Part model, mm, in its own coordinate system. A direction names the side the tool comes from. Coordinates: 2 decimals unless noted, no trailing zeros. Loops run counter-clockwise (first coordinate to the right, second up) from the corner with the lowest first, then second, coordinate; pieces in that order, holes last. Notation, with made-up numbers: (-0.5, 67.5) - (25.5, 67.5) arc R17 ccw to (25.5, 74.5) - close; hole circle Ø9 at (23.25, 54). An arc over 180 degrees is marked (long way). Use a Markdown table: item, result. Add a question column.
1) Band-saw the part on A-A (y = 2.55). Give the cut face in (x, z).
2) Band-saw the part on D-D (x = 24). Give the cut face in (y, z).
3) Pull direction X, two halves, no side cores. Call faces 4 (the face through (31, 5, -8)), 5 (the face through (67.47, 2.54, -27.45)), 6 (the face through (4.5, 2, -5)): +X half, -X half, draft (parallel to the pull), parting line (faces both ways), or undercut.
4) Band-saw the part on B-B (z = -20.5). Give the cut face in (x, y).
5) Probe probe 1 along X at (y, z) = (2.85, 0); probe 2 along X at (y, z) = (3.5, -10.5); probe 3 along X at (y, z) = (3.9, -18). List the from-to ranges inside material, lowest first. Write a range as [from, to].
6) Drop flat-ended pins along their axis: P1, Ø3, axis at x = 32, y = 3.5, coming from the -Z side; P2, Ø1, axis at x = 5.5, y = 2.5, coming from the +Z side. Give the stop position or say it passes through.
7) Band-saw the part on C-C (x = 64). Give the cut face in (y, z), plus the area to 3 significant figures.
8) Tool access for faces 1 (the face through (62.137, 2.465, 0.969)), 2 (the face through (59.5, 2, -6)), 3 (the face through (58.68, 2.46, -22.93)): list every direction of +Z, -Z, +X, -X, +Y, -Y with a clear straight run to the whole face (end or side of a thin tool).
from build123d import *

# Parameters (mm, degrees)
SKETCH1_R           = 2.1
BOSS_EXTRUDE1_DEPTH = 5
FILLET2_R           = 2


with BuildPart() as part:
    # Sketch1 → Boss-Extrude1 (new body)
    with BuildSketch(Plane(origin=(0, 0, 0), x_dir=(1, 0, 0), z_dir=(0, 1, 0))):
        with BuildLine():
            Line((68.5, 0), (68.5, 15))
            Line((68.5, 15), (68.5, 24.639286301))
            Line((68.5, 24.639286301), (68.5, 29.417680708))
            Line((68.5, 29.417680708), (51.680517538, 18.308520556))
            ThreePointArc((51.680517538, 18.308520556), (31.678817451, 11.020026075), (11.677117365, 18.308520556))
            Line((11.677117365, 18.308520556), (-4.5, 28.993402687))
            Line((-4.5, 28.993402687), (-4.5, 0))
            ThreePointArc((-4.5, 0), (0, -4.5), (4.5, 0))
            Line((4.5, 0), (4.5, 15))
            ThreePointArc((4.5, 15), (32, 5.201587921), (59.5, 15))
            Line((59.5, 15), (59.5, 0))
            ThreePointArc((59.5, 0), (64, -4.5), (68.5, 0))
        make_face()
        with Locations(Location((0, 0, 0), (0, 0, 270))):
            Circle(SKETCH1_R, mode=Mode.SUBTRACT)
        with Locations(Location((64, 0, 0), (0, 0, 270))):
            Circle(SKETCH1_R, mode=Mode.SUBTRACT)
    extrude(amount=BOSS_EXTRUDE1_DEPTH)

    # Fillet2
    fillet2_edges = [part.edges().sort_by_distance(p)[0] for p in [
        (59.5, 2.5, -15),
        (4.5, 2.5, -15),
        (-4.5, 2.5, -28.993402687),
        (11.677117365, 2.5, -18.308520556),
        (51.680517538, 2.5, -18.308520556),
        (68.5, 2.5, -29.417680708),
    ]]
    fillet(fillet2_edges, radius=FILLET2_R)


solid = part.part
Answer block:
| question | item | result |
|---|---|---|
| 1 | outline | (-4.5, -25.28) arc R2 ccw to (-1.4, -26.94) - (11.58, -18.37) arc R2 ccw to (11.76, -18.24) arc R31.09 cw to (51.6, -18.24) arc R2 ccw to (51.78, -18.37) - (65.4, -27.37) arc R2 ccw to (68.5, -25.7) - (68.5, 0) arc R4.5 ccw to (59.5, 0) - (59.5, -11.02) arc R2 cw to (56.38, -12.68) arc R43.49 ccw to (7.62, -12.68) arc R2 cw to (4.5, -11.02) - (4.5, 0) arc R4.5 ccw to (-4.5, 0) - close; hole circle Ø4.2 at (0, 0); hole circle Ø4.2 at (64, 0) |
| 2 | outline | (0, -11.98) - (5, -11.98) - (5, -5.94) - (0, -5.94) - close |
| 3 | face 4 | draft |
| 3 | face 5 | parting line |
| 3 | face 6 | undercut |
| 4 | outline | (-4.5, 0) - (8.36, 0) - (8.36, 5) - (-4.5, 5) - close; (55, 0) - (68.5, 0) - (68.5, 5) - (55, 5) - close |
| 5 | probe 1 | [-4.5, -2.1], [2.1, 4.5], [59.5, 61.9], [66.1, 68.5] |
| 5 | probe 2 | [-4.5, 4.5], [11.2, 52.8], [59.5, 68.5] |
| 5 | probe 3 | [-4.5, 12.05], [51.31, 68.5] |
| 6 | P1 | z = -11.07 |
| 6 | P2 | z = -12.34 |
| 7 | outline | (0, -26.45) - (5, -26.45) - (5, -2.1) - (0, -2.1) - close; (0, 2.1) - (5, 2.1) - (5, 4.5) - (0, 4.5) - close |
| 7 | area | 134 mm2 |
| 8 | face 1 | +Y, -Y |
| 8 | face 2 | +Z, +Y, -Y |
| 8 | face 3 | -Z, +Y, -Y |
